Read the model definition and answer for the solid it produces. Units are mm, in the model's axes. Give positions to 0.01 mm unless a question says otherwise; leave off trailing zeros. Write each loop counter-clockwise with the first axis right and the second up, starting at its lowest first coordinate (ties: lowest second). Pieces come first, ordered by that corner, then holes. Notation, with made-up numbers: (57, -9) -> (85, -9) arc R23 cw to (85, 8) -> close; hole circle Ø10 at (-8, 65.5). An arc over 180 degrees is marked (long way). Put each result on its own line as item: value. Start each with the question number.
from build123d import *

# Parameters (mm, degrees)
F0_W     = 25
F0_H     = 12.5
F1_DEPTH = 15


with BuildPart() as f1:
    # F0 (on Front) → F1 (new body)
    with BuildSketch(Plane.XZ):
        with BuildLine():
            Line((12.5, -100), (-12.5, -100))
            ThreePointArc((-12.5, -100), (0, -112.5), (12.5, -100))
        make_face()
        with BuildLine():
            ThreePointArc((12.5, -100), (0, -87.5), (-12.5, -100))
            Line((-12.5, -100), (12.5, -100))
        make_face()
        with BuildLine():
            Line((12.5, 37.5), (-12.5, 37.5))
            Line((-12.5, 37.5), (-12.5, -100))
            ThreePointArc((-12.5, -100), (0, -87.5), (12.5, -100))
            Line((12.5, -100), (12.5, 37.5))
        make_face()
        with Locations((0, 56.25)):
            Rectangle(F0_W, F0_H)
        with Locations((0, 43.75)):
            Rectangle(F0_W, F0_H)
        with BuildLine():
            Line((-12.5, 50), (-12.5, 62.5))
            Line((-12.5, 62.5), (-37.5, 62.5))
            ThreePointArc((-37.5, 62.5), (-60.4639663386, 70.3536469359), (-73.8092188707, 90.625))
            ThreePointArc((-73.8092188707, 90.625), (-89.0372918276, 99.6030729569), (-98.0153647845, 84.375))
            ThreePointArc((-98.0153647845, 84.375), (-75.773277231, 50.5894115599), (-37.5, 37.5))
            Line((-37.5, 37.5), (-12.5, 37.5))
            Line((-12.5, 37.5), (-12.5, 50))
        make_face()
        with BuildLine():
            Line((37.5, 50), (12.5, 50))
            Line((12.5, 50), (12.5, 37.5))
            Line((12.5, 37.5), (37.5, 37.5))
            ThreePointArc((37.5, 37.5), (60.4639663386, 29.6463530641), (73.8092188707, 9.375))
            ThreePointArc((73.8092188707, 9.375), (89.0372918276, 0.3969270431), (98.0153647845, 15.625))
            ThreePointArc((98.0153647845, 15.625), (75.773277231, 49.4105884401), (37.5, 62.5))
            ThreePointArc((37.5, 62.5), (46.875, 58.2679728471), (49.9019592706, 48.4375))
            ThreePointArc((49.9019592706, 48.4375), (43.75, 49.6078370825), (37.5, 50))
        make_face()
        with BuildLine():
            Line((37.5, 62.5), (12.5, 62.5))
            Line((12.5, 62.5), (12.5, 50))
            Line((12.5, 50), (37.5, 50))
            ThreePointArc((37.5, 50), (43.75, 49.6078370825), (49.9019592706, 48.4375))
            ThreePointArc((49.9019592706, 48.4375), (46.875, 58.2679728471), (37.5, 62.5))
        make_face()
        with BuildLine():
            ThreePointArc((12.5, 100), (0, 87.5), (-12.5, 100))
            Line((-12.5, 100), (-12.5, 62.5))
            Line((-12.5, 62.5), (12.5, 62.5))
            Line((12.5, 62.5), (12.5, 100))
        make_face()
        with BuildLine():
            Line((12.5, 100), (-12.5, 100))
            ThreePointArc((-12.5, 100), (0, 87.5), (12.5, 100))
        make_face()
        with BuildLine():
            ThreePointArc((12.5, 100), (0, 112.5), (-12.5, 100))
            Line((-12.5, 100), (12.5, 100))
        make_face()
    extrude(amount=-F1_DEPTH)


solid = f1.part
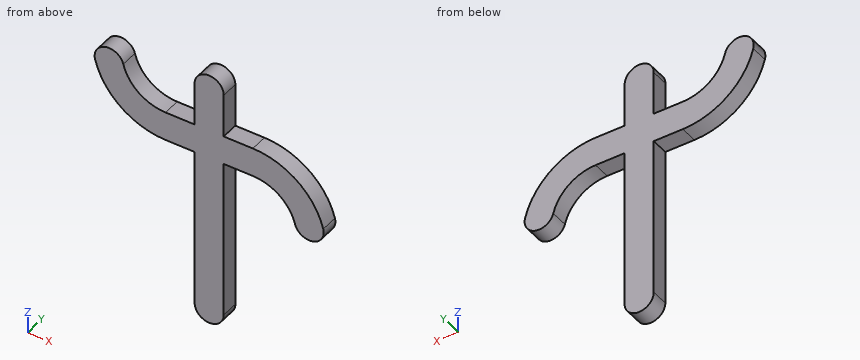
1) A cutting plane is placed at C-C on x = -21.5. Give the vertices of the cut face in (y, z).
2) A cutting plane is placed at B-B on y = 4.5. Give the vertices of the cut face in (x, z) (3 decimals), and give its area (3 significant figures).
3) Straight lines are drawn through the part: line 1 (X direction, y = 1.5, z = 13); line 2 (X direction, y = 11, z = -58); line 3 (Z direction, x = -25, y = 1). For each, find the intervals that lie inside material, in ascending order. Write a range as [from, to].
4) A cutting plane is placed at D-D on z = -78. Give the vertices of the cut face in (x, y), and give its area (3 significant figures).
5) Each of these flat-tipped pins is pushed along its axis until it touches: pin 1 Ø6 at (y, z) = (13, -30.5) entering from +X; pin 2 Ø8 at (x, y) = (7, 12) entering from +Z; pin 3 Ø4.5 at (x, y) = (29.5, 8.5) entering from -Z; pin 4 Ø12 at (x, z) = (60.5, 26) entering from +Y. Where does it stop, or does it pass through?
6) A cutting plane is placed at A-A on z = 12.5. Give the vertices of the cut face in (x, y).
Results found:
1. outline: (0, 37.5) -> (15, 37.5) -> (15, 62.5) -> (0, 62.5) -> close
2. outline: (-98.015, 84.375) arc R62.5 ccw to (-37.5, 37.5) -> (-12.5, 37.5) -> (-12.5, -100) arc R12.5 ccw to (12.5, -100) -> (12.5, 37.5) -> (37.5, 37.5) arc R37.5 cw to (73.809, 9.375) arc R12.5 ccw to (98.015, 15.625) arc R62.5 ccw to (37.5, 62.5) -> (12.5, 62.5) -> (12.5, 100) arc R12.5 ccw to (-12.5, 100) -> (-12.5, 62.5) -> (-37.5, 62.5) arc R37.5 cw to (-73.809, 90.625) arc R12.5 ccw to start
2. area: 10,500 mm²
3. line 1: x = [-12.5, 12.5], [72.67, 98.4]
3. line 2: x = [-12.5, 12.5]
3. line 3: z = [37.5, 62.5]
4. outline: (-12.5, 0) -> (12.5, 0) -> (12.5, 15) -> (-12.5, 15) -> close
4. area: 375 mm²
5. pin 1: stops at x = 12.5
5. pin 2: stops at z = 112.13
5. pin 3: stops at z = 37.5
5. pin 4: stops at y = 15
6. outline: (-12.5, 0) -> (12.5, 0) -> (12.5, 15) -> (-12.5, 15) -> close; (72.86, 0) -> (98.41, 0) -> (98.41, 15) -> (72.86, 15) -> close
